Read the model definition and answer for the solid it produces. Units are mm, in the model's axes. Face numbers are marked on the shaded views. A direction names the side the tool comes from. Coordinates: 2 decimals unless noted, no trailing zeros. Write each loop counter-clockwise with the first axis right and the second up, starting at its lowest first coordinate (ties: lowest second). Pieces come first, ordered by that corner, then holes.
1) The part is cut by section A-A (z = 15). Determine the outline of the cut face in (x, y).
2) Find the intervals of material crossed by line 1 (Y direction, x = 11.5, z = 19.75); line 2 (X direction, y = -0.5, z = 22.25); line 3 (X direction, y = 12.75, z = 7.75) (3 decimals), in increasing order.
3) Determine the mould class of the marked faces 3, 4 and 5 for opening direction Y: +Y half, -Y half, draft (parallel to the pull), parting line (faces both ways), or undercut.
4) The part is cut by section C-C (x = 18.5). Determine the outline of the cut face in (y, z).
5) The part is cut by section B-B (z = 27). Determine the outline of the cut face in (x, y), then the cut area to 3 significant figures.
6) Each of these flat-tipped pins is pushed along its axis until it touches: pin 1 Ø3 at (x, z) = (32.5, 13.5) entering from +Y; pin 2 Ø1.2 at (x, z) = (40, 14.5) entering from +Y; pin 3 Ø10 at (y, z) = (14, 11.5) entering from +X. Where does it stop, or does it pass through?
7) Which of the six approach directions +Z, -Z, +X, -X, +Y, -Y give full straight-line access (tool end or side, diameter ignored) to the marked faces 1 and 2?
8) The part is cut by section D-D (y = 8.75). Determine the outline of the cut face in (x, z), then the cut area to 3 significant figures.
Autodesk Fusion 360 part; units mm, degrees
sketch "Sketch1" plane through (0, 0, 0) normal (0, 0, 1) x (1, 0, 0)
  line L0 (0, 0) -> (36.8248, 0)
  line L1 (50, -3) -> (0, -3)
  line L2 (0, -3) -> (0, 0)
  line L3 (40.6659, 8.2009) -> (35, 15)
  line L4 (50.3841, 1.2252) -> (37.3047, 16.9206)
  line L5 (35, 15) -> (37.3047, 16.9206)
  arc A0 (50, -3) -> (50.3841, 1.2252) centre (48.0794, -0.6953) ccw
  arc A1 (36.8248, 0) -> (40.6659, 8.2009) centre (36.8248, 5) ccw
  dimension "d1" = 3
  dimension "d3" = 3
  dimension "d4" = 5
extrude "Extrude1" add sketch "Sketch1" along normal blind 30
sketch "Sketch2" plane through (0, 0, 0) normal (1, 0, 0) x (0, 1, 0)
  line L0 (0, 0) -> (0, 30)
  line L1 (0, 10) -> (25, 10)
  line L2 (0, 20) -> (25, 20)
  line L3 (11, 10) -> (11, 20)
  line L4 (20, 10) -> (20, 20)
extrude "Extrude2" cut sketch "Sketch2" along normal blind 58 contours L1 L2 L3 L4
fillet "Fillet1" radius 1.5 2 edges at (36.1523, 15.9603, 20) (36.1523, 15.9603, 10)
fillet "Fillet2" radius 1.5 2 edges at (40.2859, 11, 20) (40.2859, 11, 10)
fillet "Fillet3" radius 2 2 edges at (36.1523, 15.9603, 0) (36.1523, 15.9603, 30)
fillet "Fillet4" radius 7.5 2 edges at (0, -1.5, 0) (0, -1.5, 30)
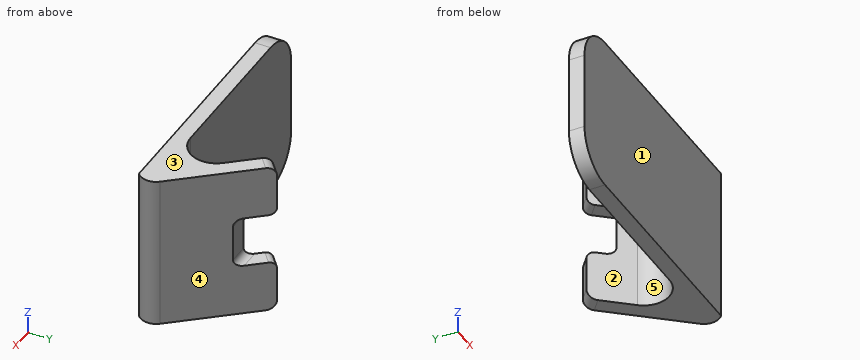
Reported:
1. outline: (0, -3) - (50, -3) arc R3 ccw to (50.38, 1.23) - (42.24, 11) - (38.33, 11) - (40.67, 8.2) arc R5 cw to (36.82, 0) - (0, 0) - close
2. line 1: y = -3 to 0
2. line 2: x = 0 to 51.07
2. line 3: x = 36.875 to 40.78
3. face 3: draft
3. face 4: +Y half
3. face 5: undercut
4. outline: (-3, 0) - (0, 0) - (0, 30) - (-3, 30) - close
5. outline: (1.5, -3) - (50, -3) arc R3 ccw to (50.38, 1.23) - (37.3, 16.92) - (35, 15) - (40.67, 8.2) arc R5 cw to (36.82, 0) - (1.5, 0) - close
5. area: 235 mm2
6. pin 1: stops at y = 0
6. pin 2: stops at y = 11
6. pin 3: stops at x = 43.91
7. face 1: +Z, -Z, +X, -X, -Y
7. face 2: +Z, -Z, -X
8. outline: (40.21, 0) - (44.11, 0) - (44.11, 30) - (40.21, 30) - close
8. area: 117 mm2
